Can you work these out from the model? Positions are in its coordinate system, mm. A direction names the side the tool comes from. Round coordinates to 2 decimals unless told otherwise and drop trailing zeros. Write each loop counter-clockwise with the first axis right and the second up, starting at its lowest first coordinate (ties: lowest second). Pieces come first, ordered by that corner, then holes. Notation, with made-up numbers: (65.5, -14) - (107.5, -14) arc R25 cw to (107.5, 14) - close; hole circle Ø9 at (-19.75, 84.25). An arc over 180 degrees is marked (long way). One line per item, written item: value. Start each with the question number.
(1) If I drill on L1, parallel to Y at x = -7.5, z = 11.75; L2, parallel to X at y = 15, z = 9.5; L3, parallel to X at y = 34.5, z = 19.25, over which ranges is the centre line in solid material (lowest first)? Write a range as from..to.
(2) I want a section at C-C on y = 9. List the corners of the cut face in (x, z) for me, plus the area to 3 significant figures.
(3) I want a section at B-B on z = 19.05. List the corners of the cut face in (x, y) for me, plus the area to 3 significant figures.
(4) I want a section at A-A on z = 3.5. List the corners of the cut face in (x, y) for me.
(5) On a 3-axis mill with a long thin cutter (end or side, diameter ignored), from which of +Z, -Z, +X, -X, +Y, -Y can I reach the whole of each face in a straight line? I mean faces 1 (the face through (-11, 13.669, 6)), 2 (the face through (-11, 7.319, 6)), 3 (the face through (-12.06, 27.75, 13.47)). Say none if no direction works.
(6) I'm going to push flat-ended pins straight in: pin 1 Ø6 at (x, z) = (-9.5, 5.5) entering from -Y; pin 2 Ø2.5 at (y, z) = (8.5, 3.5) entering from -X; pin 3 Ø1.6 at (y, z) = (8.5, 6) entering from +X. Where does each tip first touch, or does it pass through?
(7) I want a section at D-D on x = -7.5. List the corners of the cut face in (y, z) for me.
Autodesk Inventor part; units mm, degrees
ref_plane "YZ Plane" through (0, 0, 0) normal (1, 0, 0) x (0, 1, 0)
ref_plane "XZ Plane" through (0, 0, 0) normal (0, 1, 0) x (-1, 0, 0)
ref_plane "XY Plane" through (0, 0, 0) normal (0, 0, 1) x (1, 0, 0)
ref_plane "Work Plane1" through (-10.8248, 8.3603, 0) normal (0, 0, 1) x (1, 0, 0)
sketch "Sketch1" plane through (-10.8248, 8.3603, 0) normal (0, 0, 1) x (1, 0, 0)
  line L0 (-3.81, 2.1338) -> (3.81, 2.1338)
  line L1 (3.81, 2.1338) -> (3.81, 5.3088)
  line L2 (3.81, 5.3088) -> (-3.81, 5.3088)
  line L3 (-3.81, 5.3088) -> (-3.81, 2.1338)
  line L4 (3.81, -1.0412) -> (-3.81, -1.0412)
  line L5 (-3.81, -1.0412) -> (-3.81, -4.2162)
  line L6 (-3.81, -4.2162) -> (3.81, -4.2162)
  line L7 (3.81, -4.2162) -> (3.81, -1.0412)
  line L8 (3.81, -1.0412) -> (-3.81, -1.0412)
  line L9 (-3.81, -1.0412) -> (-3.81, 2.1338)
  line L10 (-3.81, 2.1338) -> (3.81, 2.1338)
  line L11 (3.81, 2.1338) -> (3.81, -1.0412)
  line L12 (3.81, 5.3088) -> (-3.81, 5.3088)
  line L13 (-3.81, 5.3088) -> (-3.81, 8.8452)
  line L14 (-3.81, 8.8452) -> (3.81, 8.8452)
  line L15 (3.81, 8.8452) -> (3.81, 5.3088)
  point P0 (10.8248, -8.3603)
extrude "Extrusion1" add sketch "Sketch1" along normal blind 12.7 contours L0 L11 L4 L9 | L13 L14 L15 L2
sketch "Sketch2" plane through (-10.8248, 8.3603, 12.7) normal (0, 0, 1) x (1, 0, 0)
  line L0 (-6.35, -1.5875) -> (6.35, -1.5875)
  line L1 (6.35, -1.5875) -> (6.35, 9.525)
  line L2 (6.35, 9.525) -> (-6.35, 9.525)
  line L3 (-6.35, 9.525) -> (-6.35, -1.5875)
  point P0 (10.8248, -8.3603)
extrude "Extrusion2" add sketch "Sketch2" along normal blind 12.7
sketch "Sketch4" plane through (-17.1748, 17.8853, 12.7) normal (0, -1, 0) x (1, 0, 0)
  circle A0 centre (6.35, 6.35) radius 5.715
  point P0 (17.1748, -12.7)
  dimension "d4" = 11.43
extrude "Extrusion3" add sketch "Sketch4" against normal blind 20
properties part number "Joint_Wheel_Connect"
Established:
1. L1: 7.32..10.49, 13.67..17.21
1. L2: -14.63..-7.01
1. L3: -16.54..-5.11
2. outline: (-17.17, 12.7) - (-14.63, 12.7) - (-14.63, 0) - (-7.01, 0) - (-7.01, 12.7) - (-4.47, 12.7) - (-4.47, 25.4) - (-17.17, 25.4) - close
2. area: 258 mm2
3. outline: (-17.17, 6.77) - (-4.47, 6.77) - (-4.47, 17.89) - (-5.11, 17.89) - (-5.11, 37.89) - (-16.54, 37.89) - (-16.54, 17.89) - (-17.17, 17.89) - close
3. area: 370 mm2
4. outline: (-14.63, 7.32) - (-7.01, 7.32) - (-7.01, 10.49) - (-14.63, 10.49) - close; (-14.63, 13.67) - (-7.01, 13.67) - (-7.01, 17.21) - (-14.63, 17.21) - close
5. face 1: -Z, +X, -X
5. face 2: -Z, +X, -X, -Y
5. face 3: +Y
6. pin 1: y = 7.32
6. pin 2: x = -14.63
6. pin 3: x = -7.01
7. outline: (6.77, 12.7) - (7.32, 12.7) - (7.32, 0) - (10.49, 0) - (10.49, 12.7) - (13.67, 12.7) - (13.67, 0) - (17.21, 0) - (17.21, 12.7) - (17.89, 12.7) - (17.89, 14.4) - (37.89, 14.4) - (37.89, 23.7) - (17.89, 23.7) - (17.89, 25.4) - (6.77, 25.4) - close
